Geometry: final body of the model. Coordinates: model frame, mm. Face numbers are marked on the shaded views. A direction names the side the tool comes from. Round coordinates to 2 decimals unless told otherwise and drop trailing zeros. Order: outer loops, then holes, each group sorted by start corner. A loop starts at its lowest first (then second) coordinate and runs counter-clockwise, first axis right, second up. Notation, with made-up numbers: M 36.25,43 L 48.25,43 A29 cw 48.25,72 Z; hole C 42,20.5 d11. An arc over 180 degrees is marked long. Put each result on its own line as item: value. Start each with the question number.
1) Section A-A, the plane x = 3. Return loops of the section in (y, z), then the cut area to 3 significant figures.
2) Section C-C, the plane y = -2. Return loops of the section in (x, z).
3) First-contact query: P1, Ø1.5, axis at x = -5, y = 5, coming from the +Z side; P2, Ø2, axis at x = 14.5, z = 11.5, coming from the -Y side; P3, Ø4, axis at x = -10, y = 15, coming from the +Z side. Flat tips, straight axial feed; report the tip coordinate or a pass-through.
4) Material intervals for probe 1 along Z at (x, y) = (-7, -5.5); probe 2 along Y at (x, z) = (14, 2.5), sorted ascending. Write a range as [from, to].
5) Access query for the marked faces 1 and 2. Directions: +Z, -Z, +X, -X, +Y, -Y. A direction counts if a zero-diameter tool reaches every point of the face in a straight line with its end or side. Return the directions, or none.
6) Section D-D, the plane x = -12.5. Return loops of the section in (y, z) (3 decimals), then the cut area to 3 significant figures.
7) Section B-B, the plane z = 12. Return loops of the section in (x, y) (3 decimals), then the cut area to 3 significant figures.
from build123d import *

# Parameters (mm, degrees)
F0_W     = 50
F0_H     = 50
F1_DEPTH = 10
F2_T     = -1
F3_R     = 3.175
F4_DEPTH = 2
F5_R     = 4.70576
F5_R_2   = 3.175
F6_DEPTH = 5
F7_R     = 1.25
F8_DEPTH = 1.5


with BuildPart() as f1:
    # F0 (on Top) → F1 (new body)
    with BuildSketch(Plane.XY):
        Rectangle(F0_W, F0_H)
    extrude(amount=F1_DEPTH)

    # F2 (hollow: no face is removed)
    offset(amount=F2_T, mode=Mode.SUBTRACT)

    # F3 (on face) → F4 (cut)
    with BuildSketch(Plane.XY.offset(10)):
        with Locations((12.5, 0)):
            Circle(F3_R)
        with Locations((-12.5, 0)):
            Circle(F3_R)
    extrude(amount=-F4_DEPTH, mode=Mode.SUBTRACT)

    # F5 (on face) → F6 (join)
    with BuildSketch(Plane.XY.offset(10)):
        with Locations((-12.5, 0)):
            Circle(F5_R)
        with Locations((-12.5, 0)):
            Circle(F5_R_2, mode=Mode.SUBTRACT)
        with Locations((12.5, 0)):
            Circle(F5_R)
        with Locations((12.5, 0)):
            Circle(F5_R_2, mode=Mode.SUBTRACT)
    extrude(amount=F6_DEPTH)

    # F7 (on face) → F8 (cut)
    with BuildSketch(Plane.XY.offset(10)):
        with BuildLine():
            ThreePointArc((-20, 18.75), (-19.1161165235, 19.1161165235), (-18.75, 20))
            ThreePointArc((-18.75, 20), (-20.8838834765, 20.8838834765), (-20, 18.75))
        make_face()
        with BuildLine():
            ThreePointArc((-18.75, -15), (-19.1161165235, -14.1161165235), (-20, -13.75))
            Line((-20, -13.75), (-20, -16.25))
            ThreePointArc((-20, -16.25), (-19.1161165235, -15.8838834765), (-18.75, -15))
        make_face()
        with BuildLine():
            Line((-20, -16.25), (-20, -13.75))
            ThreePointArc((-20, -13.75), (-21.25, -15), (-20, -16.25))
        make_face()
        with BuildLine():
            ThreePointArc((-18.75, -10), (-19.1161165235, -9.1161165235), (-20, -8.75))
            Line((-20, -8.75), (-20, -11.25))
            ThreePointArc((-20, -11.25), (-19.1161165235, -10.8838834765), (-18.75, -10))
        make_face()
        with BuildLine():
            Line((-20, -11.25), (-20, -8.75))
            ThreePointArc((-20, -8.75), (-21.25, -10), (-20, -11.25))
        make_face()
        with BuildLine():
            ThreePointArc((-18.75, -5), (-19.1161165235, -4.1161165235), (-20, -3.75))
            Line((-20, -3.75), (-20, -6.25))
            ThreePointArc((-20, -6.25), (-19.1161165235, -5.8838834765), (-18.75, -5))
        make_face()
        with BuildLine():
            Line((-20, -6.25), (-20, -3.75))
            ThreePointArc((-20, -3.75), (-21.25, -5), (-20, -6.25))
        make_face()
        with BuildLine():
            ThreePointArc((-18.75, 0), (-19.1161165235, 0.8838834765), (-20, 1.25))
            Line((-20, 1.25), (-20, -1.25))
            ThreePointArc((-20, -1.25), (-19.1161165235, -0.8838834765), (-18.75, 0))
        make_face()
        with BuildLine():
            Line((-20, -1.25), (-20, 1.25))
            ThreePointArc((-20, 1.25), (-21.25, 0), (-20, -1.25))
        make_face()
        with BuildLine():
            ThreePointArc((-18.75, 5), (-19.1161165235, 5.8838834765), (-20, 6.25))
            Line((-20, 6.25), (-20, 3.75))
            ThreePointArc((-20, 3.75), (-19.1161165235, 4.1161165235), (-18.75, 5))
        make_face()
        with BuildLine():
            Line((-20, 3.75), (-20, 6.25))
            ThreePointArc((-20, 6.25), (-21.25, 5), (-20, 3.75))
        make_face()
        with BuildLine():
            ThreePointArc((-18.75, 10), (-19.1161165235, 10.8838834765), (-20, 11.25))
            Line((-20, 11.25), (-20, 8.75))
            ThreePointArc((-20, 8.75), (-19.1161165235, 9.1161165235), (-18.75, 10))
        make_face()
        with BuildLine():
            Line((-20, 8.75), (-20, 11.25))
            ThreePointArc((-20, 11.25), (-21.25, 10), (-20, 8.75))
        make_face()
        with BuildLine():
            ThreePointArc((-18.75, 15), (-19.1161165235, 15.8838834765), (-20, 16.25))
            Line((-20, 16.25), (-20, 13.75))
            ThreePointArc((-20, 13.75), (-19.1161165235, 14.1161165235), (-18.75, 15))
        make_face()
        with BuildLine():
            Line((-20, 13.75), (-20, 16.25))
            ThreePointArc((-20, 16.25), (-21.25, 15), (-20, 13.75))
        make_face()
        with Locations((-15, 20)):
            Circle(F7_R)
        with Locations((-10, 20)):
            Circle(F7_R)
        with Locations((-5, 20)):
            Circle(F7_R)
        with Locations((0, 20)):
            Circle(F7_R)
        with Locations((5, 20)):
            Circle(F7_R)
        with Locations((10, 20)):
            Circle(F7_R)
        with Locations((15, 20)):
            Circle(F7_R)
        with Locations((20, 20)):
            Circle(F7_R)
        with Locations((-15, 15)):
            Circle(F7_R)
        with Locations((-10, 15)):
            Circle(F7_R)
        with Locations((-5, 15)):
            Circle(F7_R)
        with Locations((5, 15)):
            Circle(F7_R)
        with Locations((10, 15)):
            Circle(F7_R)
        with Locations((0, 15)):
            Circle(F7_R)
        with Locations((15, 15)):
            Circle(F7_R)
        with Locations((20, 15)):
            Circle(F7_R)
        with Locations((-15, 10)):
            Circle(F7_R)
        with Locations((-10, 10)):
            Circle(F7_R)
        with Locations((-5, 10)):
            Circle(F7_R)
        with Locations((0, 10)):
            Circle(F7_R)
        with Locations((10, 10)):
            Circle(F7_R)
        with Locations((15, 10)):
            Circle(F7_R)
        with Locations((5, 10)):
            Circle(F7_R)
        with Locations((20, 10)):
            Circle(F7_R)
        with Locations((-5, 5)):
            Circle(F7_R)
        with Locations((0, 5)):
            Circle(F7_R)
        with Locations((5, 5)):
            Circle(F7_R)
        with Locations((20, 5)):
            Circle(F7_R)
        Circle(F7_R)
        with Locations((20, 0)):
            Circle(F7_R)
        with Locations((-15, -15)):
            Circle(F7_R)
        with Locations((-10, -15)):
            Circle(F7_R)
        with Locations((-5, -15)):
            Circle(F7_R)
        with Locations((0, -15)):
            Circle(F7_R)
        with Locations((5, -15)):
            Circle(F7_R)
        with Locations((10, -15)):
            Circle(F7_R)
        with Locations((15, -15)):
            Circle(F7_R)
        with Locations((20, -15)):
            Circle(F7_R)
        with Locations((-20, -20)):
            Circle(F7_R)
        with Locations((-15, -20)):
            Circle(F7_R)
        with Locations((-10, -20)):
            Circle(F7_R)
        with Locations((-5, -20)):
            Circle(F7_R)
        with Locations((0, -20)):
            Circle(F7_R)
        with Locations((5, -20)):
            Circle(F7_R)
        with Locations((10, -20)):
            Circle(F7_R)
        with Locations((15, -20)):
            Circle(F7_R)
        with Locations((20, -20)):
            Circle(F7_R)
        with Locations((-15, -10)):
            Circle(F7_R)
        with Locations((-10, -10)):
            Circle(F7_R)
        with Locations((-5, -10)):
            Circle(F7_R)
        with Locations((0, -10)):
            Circle(F7_R)
        with Locations((5, -10)):
            Circle(F7_R)
        with Locations((10, -10)):
            Circle(F7_R)
        with Locations((15, -10)):
            Circle(F7_R)
        with Locations((20, -10)):
            Circle(F7_R)
        with Locations((-5, -5)):
            Circle(F7_R)
        with Locations((0, -5)):
            Circle(F7_R)
        with Locations((5, -5)):
            Circle(F7_R)
        with Locations((20, -5)):
            Circle(F7_R)
    extrude(amount=-F8_DEPTH, mode=Mode.SUBTRACT)


solid = f1.part
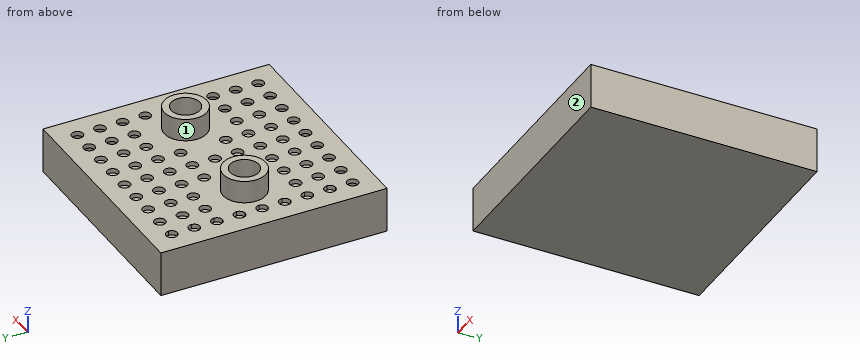
Result sheet:
1. outline: M -25,0 L 25,0 L 25,10 L -25,10 Z; hole M -24,1 L 24,1 L 24,9 L -24,9 Z
1. area: 116 mm2
2. outline: M -25,0 L 25,0 L 25,10 L 16.76,10 L 16.76,15 L 14.97,15 L 14.97,9 L 24,9 L 24,1 L -24,1 L -24,9 L -14.97,9 L -14.97,15 L -16.76,15 L -16.76,10 L -25,10 Z; M -10.03,9 L 10.03,9 L 10.03,15 L 8.24,15 L 8.24,10 L -8.24,10 L -8.24,15 L -10.03,15 Z
3. P1: stops at z = 1
3. P2: stops at y = -4.6
3. P3: stops at z = 10
4. probe 1: z = [0, 1], [9, 10]
4. probe 2: y = [-25, -24], [24, 25]
5. face 1: +Z
5. face 2: +Z, -Z, +X, -X, -Y
6. outline: M -25,0 L 25,0 L 25,10 L 4.706,10 L 4.706,15 L 3.175,15 L 3.175,9 L 24,9 L 24,1 L -24,1 L -24,9 L -3.175,9 L -3.175,15 L -4.706,15 L -4.706,10 L -25,10 Z
6. area: 125 mm2
7. outline: C -12.5,0 d9.412; C 12.5,0 d9.412; hole C -12.5,0 d6.35; hole C 12.5,0 d6.35
7. area: 75.8 mm2
